Part model, mm, in its own coordinate system. Face numbers are marked on the shaded views. A direction names the side the tool comes from. Round coordinates to 2 decimals unless told otherwise and drop trailing zeros. Write each loop counter-clockwise with the first axis right and the second up, starting at its lowest first coordinate (ties: lowest second). Pieces come first, ordered by that corner, then holes.
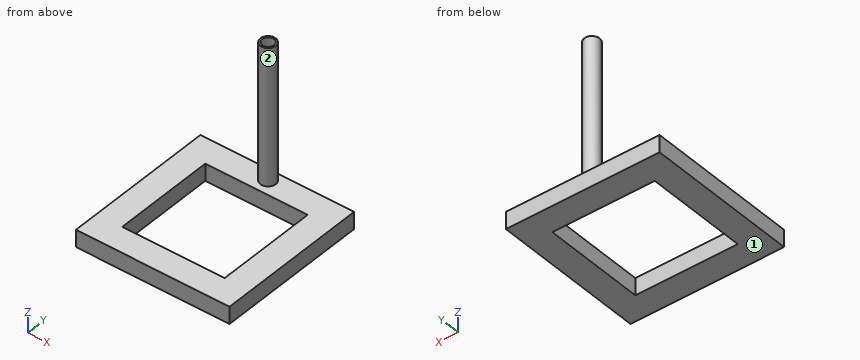
```python
from build123d import *

# Parameters (mm, degrees)
F0_W     = 90
F0_H     = 90
F1_DEPTH = 10
F2_W     = 60
F2_H     = 60
F3_DEPTH = 10
F4_R     = 4.5
F5_DEPTH = 80
F6_T     = -1


with BuildPart() as f1:
    # F0 (on Top) → F1 (new body)
    with BuildSketch(Plane.XY):
        Rectangle(F0_W, F0_H)
    extrude(amount=F1_DEPTH)

    # F2 (on face) → F3 (cut)
    with BuildSketch(Plane.XY.offset(10)):
        Rectangle(F2_W, F2_H)
    extrude(amount=-F3_DEPTH, mode=Mode.SUBTRACT)

    # F4 (on face) → F5 (join)
    with BuildSketch(Plane.XY.offset(10)):
        with Locations((0, 38.3668020368)):
            Circle(F4_R)
    extrude(amount=F5_DEPTH)

    # F6
    f6_openings = [f1.faces().sort_by_distance(p)[0] for p in [
        (0, 38.366802, 90),
    ]]
    offset(amount=F6_T, openings=f6_openings, kind=Kind.INTERSECTION)


solid = f1.part
```
Q1. Cut at A-A on y = 10. Write the cut outline in (x, z).
Values follow:
outline: (-45, 0) - (-30, 0) - (-30, 10) - (-45, 10) - close; (30, 0) - (45, 0) - (45, 10) - (30, 10) - close; hole (-44, 1) - (-31, 1) - (-31, 9) - (-44, 9) - close; hole (31, 1) - (44, 1) - (44, 9) - (31, 9) - close
Q2. Wall check: L1, parallel to Y at x = 0, z = 47.5; L2, parallel to Z at x = 36.5, y = -34; L3, parallel to X at y = 40.5, z = 70. Give the ranges that are in metal, low to high.
Values follow:
L1: y = 33.87 to 34.87, 41.87 to 42.87
L2: z = 0 to 1, 9 to 10
L3: x = -3.96 to -2.77, 2.77 to 3.96
Q3. Cut at B-B on x = 0. Write the cut outline in (y, z).
Values follow:
outline: (-45, 0) - (-30, 0) - (-30, 10) - (-45, 10) - close; (30, 0) - (45, 0) - (45, 10) - (42.87, 10) - (42.87, 90) - (41.87, 90) - (41.87, 9) - (44, 9) - (44, 1) - (31, 1) - (31, 9) - (34.87, 9) - (34.87, 90) - (33.87, 90) - (33.87, 10) - (30, 10) - close; hole (-44, 1) - (-31, 1) - (-31, 9) - (-44, 9) - close
Q4. Drop flat-ended pins along their axis: pin 1 (12 mm diameter, centred on y = 33, z = 14.5, fed in from +X); pin 2 (5 mm diameter, centred on x = -8.5, y = -31.5, fed in from +Z); pin 3 (4 mm diameter, centred on x = 0, y = 38.37, fed in from +Z). Give the stop position or say it passes through.
Values follow:
pin 1: stops at x = 45
pin 2: stops at z = 10
pin 3: stops at z = 1
Q5. Which spindle directions (+Z, -Z, +X, -X, +Y, -Y) get a long thin tool onto all of the face, cutting with end or side? Do the marked faces 1 and 2. Say none if no direction does.
Values follow:
face 1: -Z, +X, -X, +Y, -Y
face 2: +Z
Q6. Cut at D-D on x = -35. Write the cut outline in (y, z), plus the area to 3 significant figures.
Values follow:
outline: (-45, 0) - (45, 0) - (45, 10) - (-45, 10) - close; hole (-44, 1) - (44, 1) - (44, 9) - (-44, 9) - close
area: 196 mm2
